Here's the drawing with two shaded views (mm, measured from the low corner). I have some questions. Round coordinates to 2 decimals unless told otherwise and drop trailing zeros. Loops run counter-clockwise (first coordinate to the right, second up) from the corner with the lowest first, then second, coordinate; pieces in that order, holes last. Notation, with made-up numbers: M 86,41 L 108,41 A20 cw 108,78 Z; hole C 56.5,3 d6. An arc over 180 degrees is marked long. Answer as a JSON object with one key per item and string values.
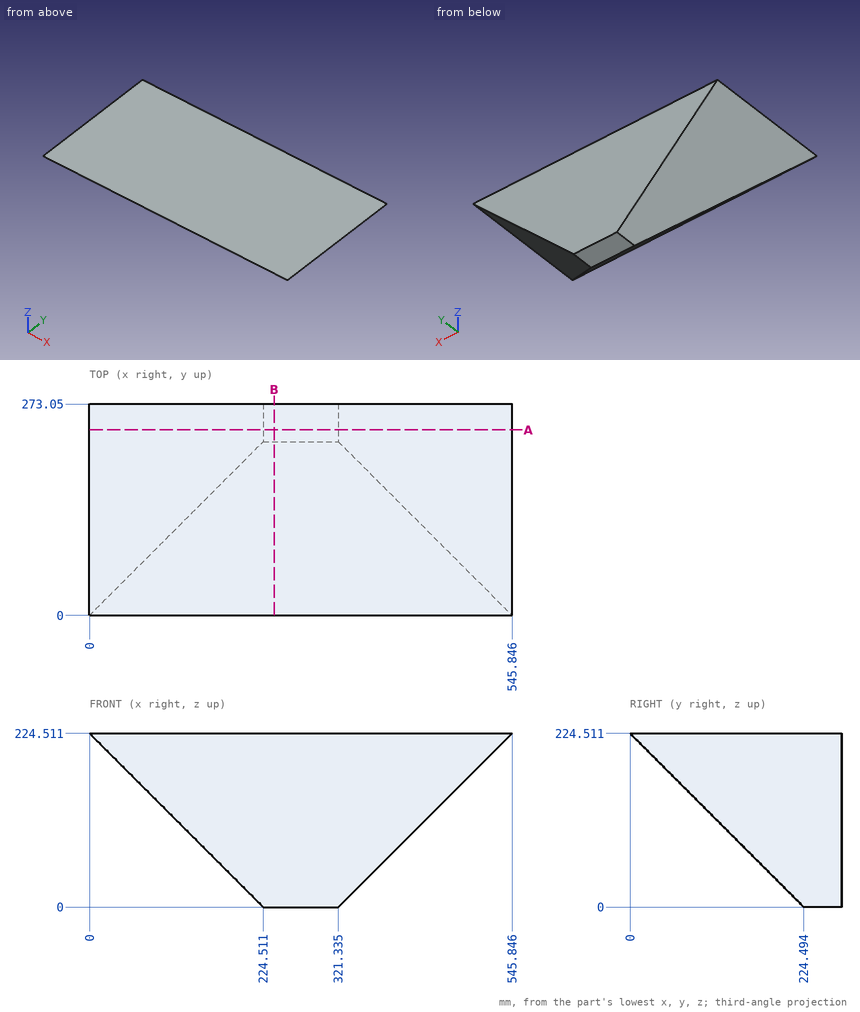
Item 1: I want a section at B-B on x = 238.5. List the corners of the cut face in (y, z) for me, plus the area to 3 significant figures.
Solution:
{"outline": "M 0,224.51 L 224.49,0 L 273.05,0 L 273.05,224.51 Z", "area": "36,100 mm2"}
Item 2: For P1, Ø4, axis at x = 256, z = 97, coming from the -Y side; P2, Ø4, axis at x = 256, y = 117.5, coming from the -Z side; P3, Ø2, axis at y = 148, z = 116, coming from the -X side, each with a flat end and sliding along its axis, tell me the tip position at first contact or that it passes through.
Solution:
{"P1": "stops at y = 125.5", "P2": "stops at z = 105", "P3": "stops at x = 107.51"}
Item 3: I want a section at A-A on y = 239.5. List the corners of the cut face in (x, z) for me (1 decimal).
Solution:
{"outline": "M 0,224.5 L 224.5,0 L 321.3,0 L 545.8,224.5 Z"}
Item 4: If I drill on L1, parallel to X at y = 219, z = 213 (1 decimal); L2, parallel to Z at x = 317.5, y = 128; L3, parallel to Z at x = 523.5, y = 112 (1 decimal), over which ranges is the centre line in solid material (lowest first)? Write a range as from..to.
Solution:
{"L1": "x = 11.5..534.3", "L2": "z = 96.5..224.51", "L3": "z = 202.2..224.5"}
